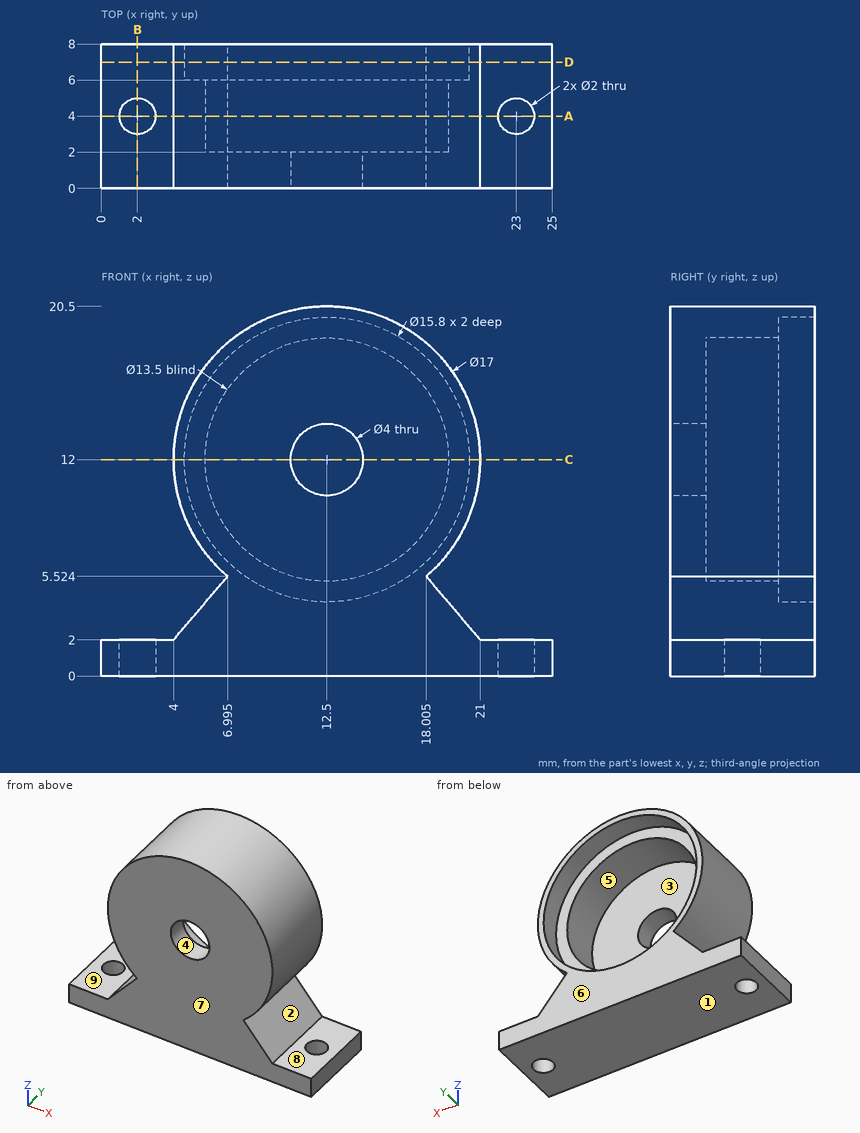
Answer from the drawing. Dimensions are ordinates in mm from the lowest x, y and z of the part. A direction names the side the tool comes from. Give positions to 0.01 mm unless a question says otherwise; leave off trailing zeros. Loops run counter-clockwise (first coordinate to the right, second up) from the corner with the lowest first, then second, coordinate; pieces in that order, holes last. Notation, with made-up numbers: (-33.5, 36.5) - (-13.5, 36.5) arc R18 ccw to (-13.5, 53.5) - close; hole circle Ø1 at (68, 43). An arc over 180 degrees is marked (long way). Answer as CSV lines item,"result". Start each with the question number.
Item 1: Each of these flat-tipped pins is pushed along its axis until it touches: pin 1 (3 mm diameter, centred on x = 24, y = 6, fed in from +Z); pin 2 (1.8 mm diameter, centred on x = 2, y = 4, fed in from -Z); pin 3 (4 mm diameter, centred on x = 15.5, y = 6.5, fed in from +Z); pin 4 (4.5 mm diameter, centred on x = 16, z = 10, fed in from +Y). Where does it stop, or does it pass through?
Item 2: Find the intervals of material crossed by line 1 (Z direction, x = 12.5, y = 0.9); line 2 (X direction, y = 3.7, z = 12); line 3 (Y direction, x = 2, z = 0.65), in increasing order. Write a range as from..to.
Item 3: A cutting plane is placed at A-A on y = 4. Count the separate pieces of the cut face and the enclosed holes in it, then the cut area to 3 significant figures.
Item 4: The mould has two halves that part along X. Classify the marked faces 1, 2, 3 and 4: +X half, -X half, draft (parallel to the pull), parting line (faces both ways), or undercut.
Item 5: A cutting plane is placed at B-B on x = 2. Determine the outline of the cut face in (y, z), then the cut area to 3 significant figures.
Item 6: A cutting plane is placed at D-D on y = 7. Determine the outline of the cut face in (x, z) (1 decimal).
Item 7: A cutting plane is placed at C-C on z = 12. Determine the outline of the cut face in (x, y).
Item 8: For the marked faces 5, 6, 7, 8 and 9, determine the directions among +Z, -Z, +X, -X, +Y, -Y from which every point of the face is accessible in a straight line to the end or side of a thin tool.
Found:
1,pin 1,"stops at z = 2"
1,pin 2,"passes through"
1,pin 3,"stops at z = 20.44"
1,pin 4,"stops at y = 2"
2,line 1,"z = 0..10, 14..20.5"
2,line 2,"x = 4..5.75, 19.25..21"
2,line 3,"y = 0..3, 5..8"
3,separate pieces,"3"
3,enclosed holes,"1"
3,area,"160 mm^2"
4,face 1,"draft"
4,face 2,"+X half"
4,face 3,"undercut"
4,face 4,"undercut"
5,outline,"(0, 0) - (3, 0) - (3, 2) - (0, 2) - close; (5, 0) - (8, 0) - (8, 2) - (5, 2) - close"
5,area,"12.0 mm^2"
6,outline,"(0, 0) - (25, 0) - (25, 2) - (21, 2) - (18, 5.5) arc R8.5 ccw (long way) to (7, 5.5) - (4, 2) - (0, 2) - close; hole circle Ø15.8 at (12.5, 12)"
7,outline,"(4, 0) - (10.5, 0) - (10.5, 2) - (5.75, 2) - (5.75, 6) - (4.6, 6) - (4.6, 8) - (4, 8) - close; (14.5, 0) - (21, 0) - (21, 8) - (20.4, 8) - (20.4, 6) - (19.25, 6) - (19.25, 2) - (14.5, 2) - close"
8,face 5,"+Y"
8,face 6,"+Z, -Z, +X, -X, +Y"
8,face 7,"+Z, -Z, +X, -X, -Y"
8,face 8,"+Z, +X, +Y, -Y"
8,face 9,"+Z, -X, +Y, -Y"
